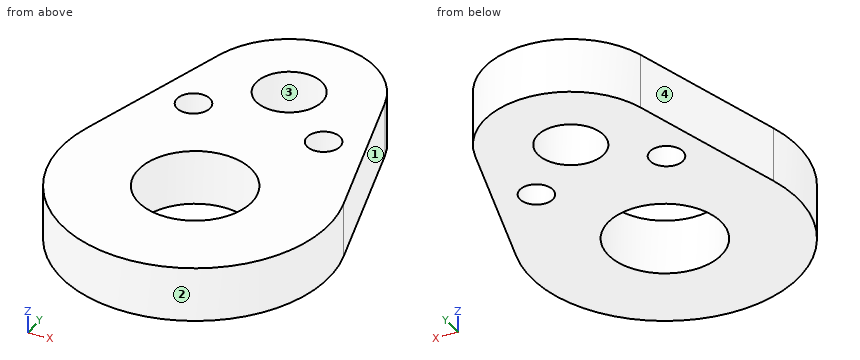
```python
from build123d import *

# Parameters (mm, degrees)
ESQUISSE1_R        = 5.129898749
ESQUISSE1_R_2      = 3
ESQUISSE1_R_3      = 1.5
BOSS_EXTRU_1_DEPTH = 5


with BuildPart() as part:
    # Esquisse1 → Boss.-Extru.1 (new body)
    with BuildSketch(Plane.XY):
        with BuildLine():
            Line((7.511654648, 17.86120118), (11.664614312, 3.334802688))
            ThreePointArc((11.664614312, 3.334802688), (0, -12.131946918), (-11.664614312, 3.334802688))
            Line((-11.664614312, 3.334802688), (-7.511654648, 17.86120118))
            ThreePointArc((-7.511654648, 17.86120118), (0, 23.526292848), (7.511654648, 17.86120118))
        make_face()
        Circle(ESQUISSE1_R, mode=Mode.SUBTRACT)
        with Locations((0, 15.713690304)):
            Circle(ESQUISSE1_R_2, mode=Mode.SUBTRACT)
        with Locations((5.904785434, 10.598001934)):
            Circle(ESQUISSE1_R_3, mode=Mode.SUBTRACT)
        with Locations((-5.904785434, 10.598001934)):
            Circle(ESQUISSE1_R_3, mode=Mode.SUBTRACT)
    extrude(amount=BOSS_EXTRU_1_DEPTH)


solid = part.part
```
Verification items for the finished model (mm, model axes). Face numbers are marked on the shaded views. Give positions to 0.01 mm unless a question says otherwise; leave off trailing zeros. Loops run counter-clockwise (first coordinate to the right, second up) from the corner with the lowest first, then second, coordinate; pieces in that order, holes last. Notation, with made-up numbers: M 62,-11 L 72,-11 A26 ccw 72,14 Z; hole C -32,0.5 d8. An arc over 180 degrees is marked long. Return JSON: item names as keys, results as strings.
1) Material ranges on L1, parallel to Y at x = 0, z = 2.55; L2, parallel to X at y = 10.5, z = 1.45; L3, parallel to Y at x = 1.75, z = 3.15, recorded low to high. Write a range as [from, to].
Findings:
{"L1": "y = [-12.13, -5.13], [5.13, 12.71], [18.71, 23.53]", "L2": "x = [-9.62, -7.4], [-4.41, 4.41], [7.4, 9.62]", "L3": "y = [-12.01, -4.82], [4.82, 13.28], [18.15, 23.33]"}
2) Gauge pin test, flat ends, axial feed: P1, Ø3, axis at y = -7.5, z = 3, coming from the +X side; P2, Ø2, axis at x = 4.5, z = 4.5, coming from the -Y side; P3, Ø3, axis at x = 3, z = 1.5, coming from the +Y side. Record the tip position at first contact, or that the pin passes through.
Findings:
{"P1": "stops at x = 10.54", "P2": "stops at y = -11.62", "P3": "stops at y = 23.38"}
3) Section check B-B, the plane y = 0. Enter the section's corners in (x, z).
Findings:
{"outline": "M -12.13,0 L -5.13,0 L -5.13,5 L -12.13,5 Z; M 5.13,0 L 12.13,0 L 12.13,5 L 5.13,5 Z"}
4) Section check A-A, the plane x = 0. Enter the section's corners in (y, z), and give its area (3 significant figures).
Findings:
{"outline": "M -12.13,0 L -5.13,0 L -5.13,5 L -12.13,5 Z; M 5.13,0 L 12.71,0 L 12.71,5 L 5.13,5 Z; M 18.71,0 L 23.53,0 L 23.53,5 L 18.71,5 Z", "area": "97.0 mm2"}
5) Section check C-C, the plane z = 1.65. Enter the section's corners in (x, y).
Findings:
{"outline": "M -11.66,3.33 A12.13 ccw long 11.66,3.33 L 7.51,17.86 A7.81 ccw -7.51,17.86 Z; hole C -5.9,10.6 d3; hole C 0,0 d10.26; hole C 0,15.71 d6; hole C 5.9,10.6 d3"}
6) Section check D-D, the plane y = 10. Enter the section's corners in (x, z), and give its area (3 significant figures).
Findings:
{"outline": "M -9.76,0 L -7.28,0 L -7.28,5 L -9.76,5 Z; M -4.53,0 L 4.53,0 L 4.53,5 L -4.53,5 Z; M 7.28,0 L 9.76,0 L 9.76,5 L 7.28,5 Z", "area": "70.1 mm2"}
7) Mould release check, pull along X, two halves, no side actions. Record for the marked faces 1, 2, 3 and 4: released by +X, released by -X, zero draft, split by the parting line, or undercut.
Findings:
{"face 1": "released by +X", "face 2": "split by the parting line", "face 3": "undercut", "face 4": "released by -X"}
